from build123d import *

# Parameters (mm, degrees)
SKETCH_R     = 11
SKETCH_R_2   = 1.5
PAD_DEPTH    = 3
SKETCH001_W  = 51
SKETCH001_H  = 3
PAD001_DEPTH = 48
POCKET_DEPTH = 5
FILLET_R     = 2
FILLET001_R  = 2


with BuildPart() as part:
    # Sketch → Pad (new body)
    with BuildSketch(Plane.XY):
        Polygon((0, 0), (51, 0), (51, 48), (48, 51), (3, 51), (0, 48), align=None)
        with Locations((25.5, 30)):
            Circle(SKETCH_R, mode=Mode.SUBTRACT)
        with Locations((10, 45.5)):
            Circle(SKETCH_R_2, mode=Mode.SUBTRACT)
        with Locations((10, 14.5)):
            Circle(SKETCH_R_2, mode=Mode.SUBTRACT)
        with Locations((41, 14.5)):
            Circle(SKETCH_R_2, mode=Mode.SUBTRACT)
        with Locations((41, 45.5)):
            Circle(SKETCH_R_2, mode=Mode.SUBTRACT)
    extrude(amount=PAD_DEPTH)

    # Sketch001 (on Face13 of Pad) → Pad001 (join)
    with BuildSketch(Plane.XY.offset(3)):
        with Locations((25.5, 1.5)):
            Rectangle(SKETCH001_W, SKETCH001_H)
    extrude(amount=PAD001_DEPTH)

    # Sketch002 (on Face18 of Pad001) → Pocket (cut)
    with BuildSketch(Plane(origin=(0, 3, 0), x_dir=(-1, 0, 0), z_dir=(0, 1, 0))):
        Polygon((-51, 48), (-51, 51), (-48, 51), align=None)
        Polygon((-3, 51), (0, 51), (0, 48), align=None)
        with BuildLine():
            ThreePointArc((-38.55959, 41), (-40.70959, 43.15), (-42.85959, 41))
            Line((-42.85959, 41), (-42.85959, 11.3))
            ThreePointArc((-42.85959, 11.3), (-40.70959, 9.15), (-38.55959, 11.3))
            Line((-38.55959, 41), (-38.55959, 11.3))
        make_face()
        with BuildLine():
            ThreePointArc((-8.55959, 40.561928), (-10.70959, 42.711928), (-12.85959, 40.561928))
            Line((-12.85959, 40.561928), (-12.85959, 11.3))
            ThreePointArc((-12.85959, 11.3), (-10.70959, 9.15), (-8.55959, 11.3))
            Line((-8.55959, 40.561928), (-8.55959, 11.3))
        make_face()
    extrude(amount=-POCKET_DEPTH, mode=Mode.SUBTRACT)

    # Fillet
    fillet_edges = [part.edges().sort_by_distance(p)[0] for p in [
        (25.5, 3, 3),
    ]]
    fillet(fillet_edges, radius=FILLET_R)

    # Fillet001
    fillet001_edges = [part.edges().sort_by_distance(p)[0] for p in [
        (25.5, 0, 0),
    ]]
    fillet(fillet001_edges, radius=FILLET001_R)


solid = part.part
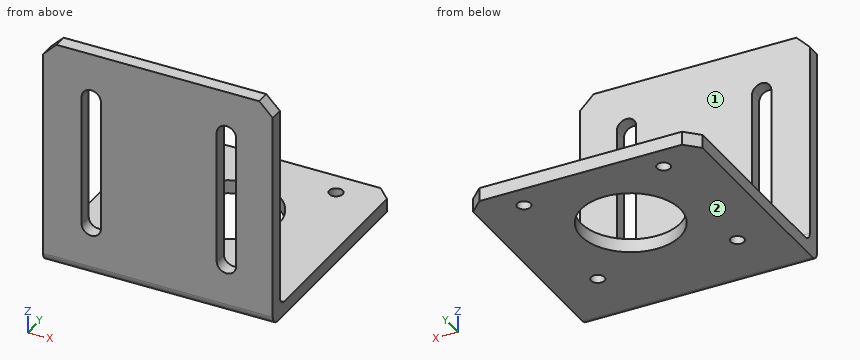
Verification items for the finished model (mm, model axes). Face numbers are marked on the shaded views. A direction names the side the tool comes from. Give positions to 0.01 mm unless a question says otherwise; leave off trailing zeros. Order: outer loops, then holes, each group sorted by start corner. A loop starts at its lowest first (then second) coordinate and runs counter-clockwise, first axis right, second up. Notation, with made-up numbers: M 11.5,-32 L 16.5,-32 A21 cw 16.5,-5 Z; hole C 19.25,-22.75 d1. An arc over 180 degrees is marked long. Answer as a JSON object with one key per item and string values. Group by question number.
1) Access from +Z, -Z, +X, -X, +Y, -Y to the whole of each face (thin tool, end or side, straight path). Record for the marked faces 1 and 2.
2) Cross-section at A-A (y = 30). Enter the section's corners in (x, z), then the cut area to 3 significant figures.
3) Cross-section at B-B (x = 25.5). Enter the section's corners in (y, z).
4) Cross-section at C-C (z = 12.5). Enter the section's corners in (x, y).
5) Scan lines: line 1 along Y through (x, z) = (10, 1.9); line 2 along Y through (x, z) = (41, 1.15); line 3 along X through (y, z) = (14, 1). Record each from-to range of solid material in increasing order. Write a range as [from, to].
6) Cross-section at D-D (y = 45.5). Enter the section's corners in (x, z).
7) Depth check by flat-ended pin: pin 1 Ø4 at (x, z) = (44, 18) entering from +Y; pin 2 Ø2.5 at (x, y) = (41, 45.5) entering from -Z; pin 3 Ø5 at (x, y) = (10, 14.5) entering from +Z. Enter the tip coordinate at first touch or a pass-through.
Result sheet:
{
 "1": {"face 1": "+Z, +X, -X, +Y", "face 2": "-Z, +X, -X, +Y, -Y"},
 "2": {"outline": "M 0,0 L 14.5,0 L 14.5,3 L 0,3 Z; M 36.5,0 L 51,0 L 51,3 L 36.5,3 Z", "area": "87.0 mm2"},
 "3": {"outline": "M 0,2 A2 ccw 2,0 L 19,0 L 19,3 L 5,3 A2 cw 3,5 L 3,51 L 0,51 Z; M 41,0 L 51,0 L 51,3 L 41,3 Z"},
 "4": {"outline": "M 0,0 L 8.56,0 L 8.56,3 L 0,3 Z; M 12.86,0 L 38.56,0 L 38.56,3 L 12.86,3 Z; M 42.86,0 L 51,0 L 51,3 L 42.86,3 Z"},
 "5": {"line 1": "y = [0, 13], [16, 44], [47, 51]", "line 2": "y = [0.19, 13], [16, 44], [47, 51]", "line 3": "x = [0, 8.59], [11.41, 39.59], [42.41, 51]"},
 "6": {"outline": "M 0,0 L 8.5,0 L 8.5,3 L 0,3 Z; M 11.5,0 L 39.5,0 L 39.5,3 L 11.5,3 Z; M 42.5,0 L 51,0 L 51,3 L 42.5,3 Z"},
 "7": {"pin 1": "stops at y = 3", "pin 2": "passes through", "pin 3": "stops at z = 3"}
}
